```python
from build123d import *

# Parameters (mm, degrees)
SKETCH_1_W         = 42
SKETCH_1_H         = 42
EXTRUDE_1_DEPTH    = 48
FILLET_1_R         = 10
SKETCH_2_R         = 11
EXTRUDE_2_DEPTH    = 2.5
SKETCH_3_R         = 3.75
EXTRUDE_3_DEPTH    = 15
HOLE_WIZARD_M4_1_D = 3.3


with BuildPart() as part:
    # 草图1 → 凸台-拉伸1 (new body)
    with BuildSketch(Plane.XY):
        with Locations((-24.739017766, 0.699593909)):
            Rectangle(SKETCH_1_W, SKETCH_1_H)
    extrude(amount=EXTRUDE_1_DEPTH)

    # 圆角1
    fillet_1_edges = [part.edges().sort_by_distance(p)[0] for p in [
        (-45.739017766, 21.699593909, 24),
        (-3.739017766, 21.699593909, 24),
        (-3.739017766, -20.300406091, 24),
        (-45.739017766, -20.300406091, 24),
    ]]
    fillet(fillet_1_edges, radius=FILLET_1_R)

    # 草图2 → 凸台-拉伸2 (add)
    with BuildSketch(Plane.XY.offset(48)):
        with Locations((-24.739017766, 0.699593909)):
            Circle(SKETCH_2_R)
    extrude(amount=EXTRUDE_2_DEPTH)

    # 草图3 → 凸台-拉伸3 (add)
    with BuildSketch(Plane.XY.offset(50.5)):
        with Locations((-24.739017766, 0.699593909)):
            Circle(SKETCH_3_R)
    extrude(amount=EXTRUDE_3_DEPTH)

    # M4 螺纹孔1 (through all)
    with Locations(Plane(origin=(0, 0, 0), x_dir=(-1, 0, 0), z_dir=(0, 0, -1))):
        with Locations((9.239017766, 16.699593909), (9.239017766, -15.300406091), (39.239017766, -15.300406091), (39.239017766, 16.699593909)):
            Hole(HOLE_WIZARD_M4_1_D / 2)


solid = part.part
```
The listing builds one solid part. Answer for the finished solid, in the listing's coordinates (mm). A direction names the side the tool comes from. Give positions to 0.01 mm unless a question says otherwise; leave off trailing zeros. Loops run counter-clockwise (first coordinate to the right, second up) from the corner with the lowest first, then second, coordinate; pieces in that order, holes last. Notation, with made-up numbers: (4.25, -21) - (18.25, -21) arc R10 ccw to (18.25, -6) - close; hole circle Ø2 at (-0.5, 68.25). An arc over 180 degrees is marked (long way). Answer as CSV lines item,"result". Start each with the question number.
Item 1: Each of these flat-tipped pins is pushed along its axis until it touches: pin 1 (6 mm diameter, centred on x = -31.5, y = -1.5, fed in from +Z); pin 2 (2 mm diameter, centred on x = -9.24, y = -15.3, fed in from +Z); pin 3 (3 mm diameter, centred on y = -13.5, z = 33.5, fed in from -X); pin 4 (6 mm diameter, centred on x = -14.5, y = 11.5, fed in from +Z). Where does it stop, or does it pass through?
Item 2: A cutting plane is placed at C-C on x = -27. Determine the outline of the cut face in (y, z).
Item 3: For faces 5 (the face through (-25, 1, 0)), 6 (the face through (-34, -8, 48)), determine the directions among +Z, -Z, +X, -X, +Y, -Y from which every point of the face is accessible in a straight line to the end or side of a thin tool.
Item 4: Find the intervals of material crossed by line 1 (Y direction, x = -10, z = 21); line 2 (X direction, y = -14, z = 41.5); line 3 (Z direction, x = -24.5, y = 11), in increasing order. Write a range as from..to.
Item 5: A cutting plane is placed at B-B on z = 18.5. Determine the outline of the cut face in (x, y).
Item 6: A cutting plane is placed at A-A on y = 6.5. Determine the outline of the cut face in (x, z).
Item 7: The mould has two halves that part along Y. Classify faces 1 (the face through (-40.887, 16.772, 24.336)), 2 (the face through (-40.887, -15.228, 24.336)), 3 (the face through (-25, 1, 65.5)), 4 (the face through (-14.578, -3.513, 49.232)): +Y half, -Y half, draft (parallel to the pull), parting line (faces both ways), or undercut.
Item 8: A cutting plane is placed at D-D on x = -32.5. Determine the outline of the cut face in (y, z).
Found:
1,pin 1,"stops at z = 50.5"
1,pin 2,"passes through"
1,pin 3,"stops at x = -45.59"
1,pin 4,"stops at z = 48"
2,outline,"(-20.3, 0) - (21.7, 0) - (21.7, 48) - (11.46, 48) - (11.46, 50.5) - (3.69, 50.5) - (3.69, 65.5) - (-2.29, 65.5) - (-2.29, 50.5) - (-10.07, 50.5) - (-10.07, 48) - (-20.3, 48) - close"
3,face 5,"-Z, +X, -X, +Y, -Y"
3,face 6,"+Z"
4,line 1,"y = -19.58..-16.76, -13.84..15.24, 18.16..20.97"
4,line 2,"x = -45.03..-40.25, -38.22..-10.25, -8.22..-4.45"
4,line 3,"z = 0..50.5"
5,outline,"(-45.74, -10.3) arc R10 ccw to (-35.74, -20.3) - (-13.74, -20.3) arc R10 ccw to (-3.74, -10.3) - (-3.74, 11.7) arc R10 ccw to (-13.74, 21.7) - (-35.74, 21.7) arc R10 ccw to (-45.74, 11.7) - close; hole circle Ø3.3 at (-39.24, -15.3); hole circle Ø3.3 at (-39.24, 16.7); hole circle Ø3.3 at (-9.24, -15.3); hole circle Ø3.3 at (-9.24, 16.7)"
6,outline,"(-45.74, 0) - (-3.74, 0) - (-3.74, 48) - (-15.39, 48) - (-15.39, 50.5) - (-34.09, 50.5) - (-34.09, 48) - (-45.74, 48) - close"
7,face 1,"undercut"
7,face 2,"undercut"
7,face 3,"draft"
7,face 4,"parting line"
8,outline,"(-20.3, 0) - (21.7, 0) - (21.7, 48) - (8.49, 48) - (8.49, 50.5) - (-7.1, 50.5) - (-7.1, 48) - (-20.3, 48) - close"
